Check sheet for the modelled part. Datum: model origin and axes. Units: mm. Give positions to 0.01 mm unless a question says otherwise; leave off trailing zeros. Write each loop counter-clockwise with the first axis right and the second up, starting at its lowest first coordinate (ties: lowest second). Pieces come first, ordered by that corner, then holes. Notation, with made-up numbers: (62.25, 86) -> (116.25, 86) arc R34 ccw to (116.25, 124) -> close; hole circle Ø5 at (53, 36.5). An arc over 180 degrees is marked (long way). Return JSON: item names as keys, results as strings.
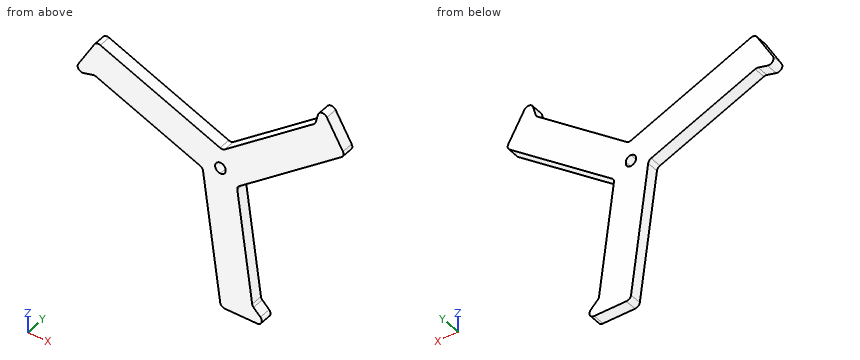
from build123d import *

# Parameters (mm, degrees)
BOSS_EXTRUDE1_DEPTH = 6.35
FILLET1_R           = 2.54


with BuildPart() as part:
    # Sketch2 → Boss-Extrude1 (new body)
    with BuildSketch(Plane(origin=(0, 0, 0), x_dir=(1, 0, 0), z_dir=(0, 1, 0))):
        Polygon((0, 76.2), (25.4, 76.2), (16.813378089, 67.613378089), (8.597359078, 6.114164014), (65.991135768, -38.1), (53.291135768, -60.097045256), (50.148214016, -48.367501593), (0.99634182, -10.502613374), (-65.991135768, -38.1), (-78.691135768, -16.102954744), (-66.961592105, -19.245876496), (-9.593700898, 4.38844936), align=None)
        with BuildLine():
            Line((2.499994, 1.658310586), (2.499994, -1.658310586))
            ThreePointArc((2.499994, -1.658310586), (-2.999994, 0), (2.499994, 1.658310586))
        make_face(mode=Mode.SUBTRACT)
    extrude(amount=BOSS_EXTRUDE1_DEPTH)

    # Fillet1
    fillet1_edges = [part.edges().sort_by_distance(p)[0] for p in [
        (-65.991135768, 3.175, 38.1),
        (-78.691135768, 3.175, 16.102954744),
        (-66.961592105, 3.175, 19.245876496),
        (-9.593700898, 3.175, -4.38844936),
        (0, 3.175, -76.2),
        (25.4, 3.175, -76.2),
        (16.813378089, 3.175, -67.613378089),
        (8.597359078, 3.175, -6.114164014),
        (65.991135768, 3.175, 38.1),
        (53.291135768, 3.175, 60.097045256),
        (50.148214016, 3.175, 48.367501593),
        (0.99634182, 3.175, 10.502613374),
        (2.499994, 3.175, 1.658310586),
        (2.499994, 3.175, -1.658310586),
    ]]
    fillet(fillet1_edges, radius=FILLET1_R)


solid = part.part
(1) Cross-section at D-D on x = -29.5. Enter the section's corners in (y, z), then the cut area to 3 significant figures.
Reply:
{"outline": "(0, 3.81) -> (6.35, 3.81) -> (6.35, 23.07) -> (0, 23.07) -> close", "area": "122 mm^2"}
(2) Depth check by flat-ended pin: pin 1 Ø3 at (x, y) = (-3, 5) entering from +Z; pin 2 Ø2 at (x, y) = (-41.5, 3.5) entering from -Z; pin 3 Ø0.7 at (y, z) = (3.5, 0) entering from -X; pin 4 Ø12 at (x, z) = (18, -52.5) entering from +Y. Enter the tip coordinate at first touch or a pass-through.
Reply:
{"pin 1": "z = 12.77", "pin 2": "z = 8.34", "pin 3": "x = -21.1", "pin 4": "y = 6.35"}
(3) Thickness scan on L1, parallel to X at y = 4, z = 22.5; L2, parallel to Z at x = 8, y = 1; L3, parallel to X at y = 0.5, z = 8. Record the ranges inside material, lowest first.
Reply:
{"L1": "-75 to -28.13, 16.57 to 45.74", "L2": "-76.2 to 15.9", "L3": "-39.66 to 26.92"}
(4) Cross-section at B-B on y = 1.75. Enter the section's corners in (x, z), then the cut area to 3 significant figures.
Reply:
{"outline": "(-75.63, 21.41) arc R2.54 ccw to (-72.77, 17.69) -> (-67.79, 19.02) arc R2.54 cw to (-66.17, 18.92) -> (-10.95, -3.83) arc R2.54 cw to (-9.4, -5.84) -> (-0.29, -74) arc R2.54 ccw to (2.22, -76.2) -> (19.27, -76.2) arc R2.54 ccw to (21.06, -71.86) -> (17.42, -68.22) arc R2.54 cw to (16.7, -66.76) -> (8.79, -7.57) arc R2.54 cw to (9.76, -5.22) -> (64.23, 36.74) arc R2.54 ccw to (64.88, 40.03) -> (56.36, 54.79) arc R2.54 ccw to (51.7, 54.17) -> (50.37, 49.2) arc R2.54 cw to (49.47, 47.84) -> (2.16, 11.4) arc R2.54 cw to (-0.36, 11.06) -> (-63.94, 37.25) arc R2.54 ccw to (-67.1, 36.17) -> close; hole (-0.26, -2.99) arc R2.54 ccw to (2.5, -0.46) -> (2.5, 0.46) arc R2.54 ccw to (-0.26, 2.99) arc R3 ccw to start", "area": "4,010 mm^2"}
(5) Cross-section at A-A on z = 29. Enter the section's corners in (x, y), then the cut area to 3 significant figures.
Reply:
{"outline": "(-71.25, 0) -> (-43.9, 0) -> (-43.9, 6.35) -> (-71.25, 6.35) -> close; (25.01, 0) -> (54.18, 0) -> (54.18, 6.35) -> (25.01, 6.35) -> close", "area": "359 mm^2"}
(6) Cross-section at C-C on z = 13. Enter the section's corners in (x, y).
Reply:
{"outline": "(-51.8, 0) -> (-5.07, 0) -> (-5.07, 6.35) -> (-51.8, 6.35) -> close; (4.24, 0) -> (33.41, 0) -> (33.41, 6.35) -> (4.24, 6.35) -> close"}
